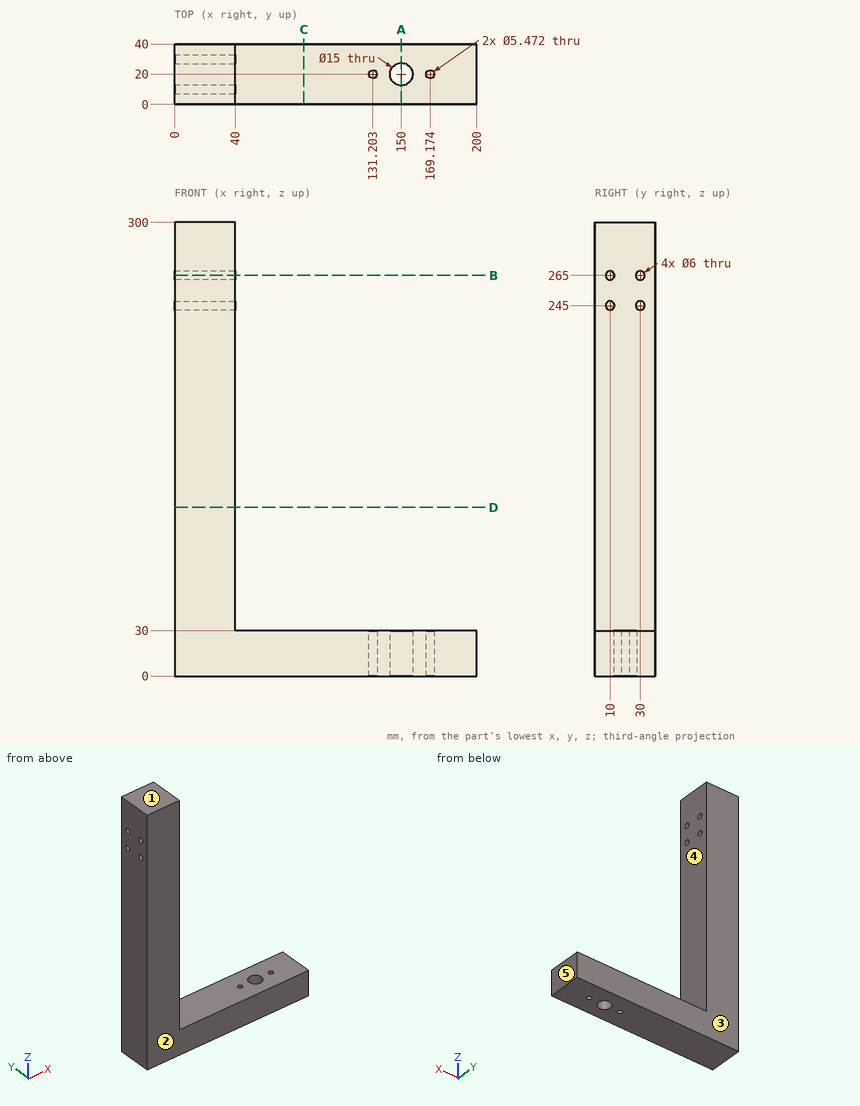
Print and shaded views of the part. All mm, measured from the part's lowest x, y and z. A direction names the side the tool comes from. Round coordinates to 2 decimals unless told otherwise and drop trailing zeros. Loops run counter-clockwise (first coordinate to the right, second up) from the corner with the lowest first, then second, coordinate; pieces in that order, holes last. Notation, with made-up numbers: (74, 81) -> (105, 81) arc R33 cw to (105, 110) -> close; hole circle Ø7 at (-13, 26). An arc over 180 degrees is marked (long way). Use CSV: the item, a comma, the result in double quotes. Start each with the question number.
1) Cut at B-B, the plane z = 265. Write the cut outline in (x, y).
2) Cut at A-A, the plane x = 150. Write the cut outline in (y, z), plus the area to 3 significant figures.
3) Pull direction Y, two halves, no side cores. Call the marked faces 1, 2 and 3: +Y half, -Y half, draft (parallel to the pull), parting line (faces both ways), or undercut.
4) Drop flat-ended pins along their axis: P1, Ø3, axis at y = 28, z = 33.5, coming from the +X side; P2, Ø3, axis at x = 147.5, y = 5, coming from the +Z side. Give the stop position or say it passes through.
5) Wall check: L1, parallel to Y at x = 32, z = 265; L2, parallel to Y at x = 150, z = 14.25; L3, parallel to Z at x = 128, y = 5.5. Give the ranges that are in metal, low to high. Write a range as [from, to].
6) Cut at C-C, the plane x = 85.5. Write the cut outline in (y, z).
7) Cut at D-D, the plane z = 111.5. Write the cut outline in (x, y), plus the area to 3 significant figures.
8) Which spindle directions (+Z, -Z, +X, -X, +Y, -Y) get a long thin tool onto all of the face, cutting with end or side? Do the marked faces 4 and 5. Say none if no direction does.
Determined:
1,outline,"(0, 0) -> (40, 0) -> (40, 7) -> (0, 7) -> close; (0, 13) -> (40, 13) -> (40, 27) -> (0, 27) -> close; (0, 33) -> (40, 33) -> (40, 40) -> (0, 40) -> close"
2,outline,"(0, 0) -> (12.5, 0) -> (12.5, 30) -> (0, 30) -> close; (27.5, 0) -> (40, 0) -> (40, 30) -> (27.5, 30) -> close"
2,area,"750 mm2"
3,face 1,"draft"
3,face 2,"-Y half"
3,face 3,"+Y half"
4,P1,"stops at x = 40"
4,P2,"stops at z = 30"
5,L1,"y = [0, 7], [13, 27], [33, 40]"
5,L2,"y = [0, 12.5], [27.5, 40]"
5,L3,"z = [0, 30]"
6,outline,"(0, 0) -> (40, 0) -> (40, 30) -> (0, 30) -> close"
7,outline,"(0, 0) -> (40, 0) -> (40, 40) -> (0, 40) -> close"
7,area,"1,600 mm2"
8,face 4,"+Z, +X, +Y, -Y"
8,face 5,"+Z, -Z, +X, +Y, -Y"
